from build123d import *

# Parameters (mm, degrees)
SKIZZE1_R                       = 3
AUFSATZ_LINEAR_AUSTRAGEN1_DEPTH = 7.25
AUFSATZ_LINEAR_START            = 5
SKIZZE3_R                       = 3.5
AUFSATZ_LINEAR_AUSTRAGEN2_DEPTH = 1
SKIZZE2_W                       = 2.6
SKIZZE2_H                       = 2.6
SCHNITT_LINEAR_AUSTRAGEN1_DEPTH = 2.5


with BuildPart() as part:
    # Skizze1 → Aufsatz-Linear austragen1 (new body)
    with BuildSketch(Plane(origin=(0, 0, 0), x_dir=(1, 0, 0), z_dir=(0, 1, 0))):
        with Locations(Location((0, 0, 0), (0, 0, 90))):
            Circle(SKIZZE1_R)
    extrude(amount=AUFSATZ_LINEAR_AUSTRAGEN1_DEPTH)

    # Skizze3 → Aufsatz-Linear austragen2 (add)
    with BuildSketch(Plane(origin=(0, 0, 0), x_dir=(1, 0, 0), z_dir=(0, 1, 0)).offset(AUFSATZ_LINEAR_START)):
        with Locations(Location((0, 0, 0), (0, 0, 270))):
            Circle(SKIZZE3_R)
    extrude(amount=AUFSATZ_LINEAR_AUSTRAGEN2_DEPTH)

    # Skizze2 → Schnitt-Linear austragen1 (cut)
    with BuildSketch(Plane(origin=(0, 7.25, 0), x_dir=(1, 0, 0), z_dir=(0, 1, 0))):
        Rectangle(SKIZZE2_W, SKIZZE2_H)
    extrude(amount=-SCHNITT_LINEAR_AUSTRAGEN1_DEPTH, mode=Mode.SUBTRACT)


solid = part.part
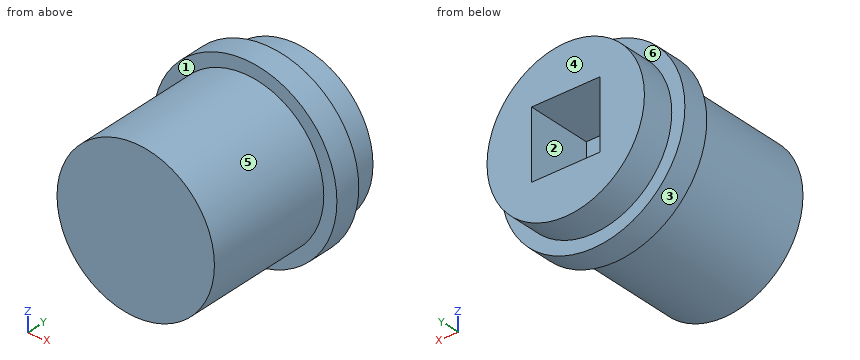
Can you work these out from the model? Positions are in its coordinate system, mm. Face numbers are marked on the shaded views. A direction names the side the tool comes from. Round coordinates to 2 decimals unless told otherwise and drop trailing zeros. Loops run counter-clockwise (first coordinate to the right, second up) from the corner with the lowest first, then second, coordinate; pieces in that order, holes last. Notation, with made-up numbers: (-21, 22.25) - (5, 22.25) arc R9 cw to (5, 34.25) - close; hole circle Ø10 at (-30.5, -8). An arc over 180 degrees is marked (long way). Answer in a Markdown table with one row per item. Add a question column.
Q1. I need wall thicknesses on L1, parallel to Y at x = 0.5, z = -0.5; L2, parallel to Z at x = -0.5, y = 6.25; L3, parallel to Y at x = -2.5, z = -1.75. Which ranges of each line are inside material? Lowest first, please.
Q2. I want a section at B-B on z = 0. List the corners of the cut face in (x, y) for me.
Q3. I want a section at C-C on y = 6.5. List the corners of the cut face in (x, z) for me.
Q4. I want a section at A-A on x = 0. List the corners of the cut face in (y, z) for me, and give its area (3 significant figures).
Q5. For pin 1 Ø1.5 at (y, z) = (2, -0.5) entering from +X; pin 2 Ø0.8 at (x, z) = (0.5, -0.5) entering from +Y; pin 3 Ø2 at (y, z) = (1.5, 2) entering from +X, each with a flat end and sliding along its axis, tell me the tip position at first contact or that it passes through.
Q6. I want a section at D-D on y = 2.75. List the corners of the cut face in (x, z) for me.
Q7. We'd pull the mould along Z, two halves only. Please class the marked faces 1, 2 and 3: pulls with the +Z half, pulls with the -Z half, needs draft (parallel to the pull), parting line crosses it, or undercut.
Q8. Which directions (+Z, -Z, +X, -X, +Y, -Y) give clear straight access to the entire face, cutting with the end or side of a thin tool? Please do the marked faces 4, 5 and 6.
A:
| question | item | result |
|---|---|---|
| 1 | L1 | 0 to 4.75 |
| 1 | L2 | -2.96 to -1.3, 1.3 to 2.96 |
| 1 | L3 | 5 to 6 |
| 2 | outline | (-3.5, 5) - (-3, 5) - (-3, 0) - (3, 0) - (3, 5) - (3.5, 5) - (3.5, 6) - (3, 6) - (3, 7.25) - (1.3, 7.25) - (1.3, 4.75) - (-1.3, 4.75) - (-1.3, 7.25) - (-3, 7.25) - (-3, 6) - (-3.5, 6) - close |
| 3 | outline | circle Ø6 at (0, 0); hole (-1.3, -1.3) - (1.3, -1.3) - (1.3, 1.3) - (-1.3, 1.3) - close |
| 4 | outline | (0, -3) - (5, -3) - (5, -3.5) - (6, -3.5) - (6, -3) - (7.25, -3) - (7.25, -1.3) - (4.75, -1.3) - (4.75, 1.3) - (7.25, 1.3) - (7.25, 3) - (6, 3) - (6, 3.5) - (5, 3.5) - (5, 3) - (0, 3) - close |
| 4 | area | 38.0 mm^2 |
| 5 | pin 1 | x = 3 |
| 5 | pin 2 | y = 4.75 |
| 5 | pin 3 | x = 2.83 |
| 6 | outline | circle Ø6 at (0, 0) |
| 7 | face 1 | needs draft |
| 7 | face 2 | undercut |
| 7 | face 3 | parting line crosses it |
| 8 | face 4 | +Z, -Z, +X, -X, +Y |
| 8 | face 5 | -Y |
| 8 | face 6 | +Y |
